Geometry check sheet. Reference: drawing and pictorial views, mm from the part's lowest x, y, z. A direction names the side the tool comes from. Give positions to 0.01 mm unless a question says otherwise; leave off trailing zeros. Write each loop counter-clockwise with the first axis right and the second up, starting at its lowest first coordinate (ties: lowest second). Pieces come first, ordered by that corner, then holes. Notation, with made-up numbers: M -29,70 L 30,70 A32 ccw 30,107 Z; hole C 1.25,-1 d11. An arc over 180 degrees is marked long. Write item = value, one per line. Start each with the question number.
1) Cross-section at A-A, the plane z = 10.25. Record the cut outline in (x, y) (3 decimals), plus the area to 3 significant figures.
2) Scan lines: line 1 along X through (y, z) = (7.25, 8); line 2 along Y through (x, z) = (7.5, 16.75); line 3 along X through (y, z) = (21.5, 6). Record each from-to range of solid material in increasing order. Write a range as [from, to].
3) Access from +Z, -Z, +X, -X, +Y, -Y to the whole of each face (thin tool, end or side, straight path). Record for the marked faces 4, 5 and 6.
4) Cross-section at B-B, the plane x = 12.5. Record the cut outline in (y, z), plus the area to 3 significant figures.
5) Mould release check, pull along X, two halves, no side actions. Record for the marked faces 1, 2 and 3: released by +X, released by -X, zero draft, split by the parting line, or undercut.
6) Cross-section at C-C, the plane y = 8.25. Give the number of separate pieces and of enclosed holes in the cut face, plus the area to 3 significant figures.
7) Go/stop test with flat-tipped pins: pin 1 (1.5 mm diameter, centred on y = 6, z = 15, fed in from -X); pin 2 (2 mm diameter, centred on y = 16.5, z = 8.5, fed in from -X); pin 3 (3 mm diameter, centred on y = 18.5, z = 5, fed in from -X). Record where each tip stops, or that it passes through.
8) Cross-section at D-D, the plane z = 4. Record the cut outline in (x, y) (3 decimals), plus the area to 3 significant figures.
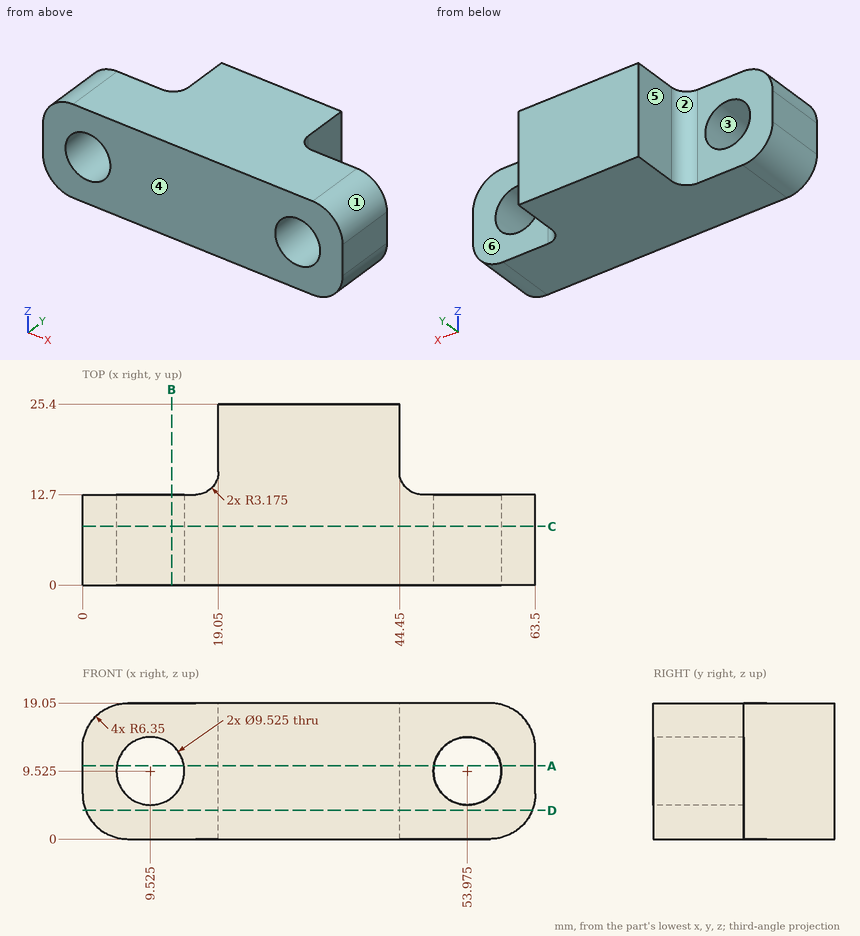
Reply:
q1.outline = M 0,0 L 4.818,0 L 4.818,12.7 L 0,12.7 Z; M 14.232,0 L 49.268,0 L 49.268,12.7 L 47.625,12.7 A3.175 cw 44.45,15.875 L 44.45,25.4 L 19.05,25.4 L 19.05,15.875 A3.175 cw 15.875,12.7 L 14.232,12.7 Z; M 58.682,0 L 63.5,0 L 63.5,12.7 L 58.682,12.7 Z
q1.area = 894 mm2
q2.line_1 = [0, 5.01], [14.04, 49.46], [58.49, 63.5]
q2.line_2 = [0, 12.7]
q2.line_3 = [19.05, 44.45]
q3.face_4 = +Z, -Z, +X, -X, -Y
q3.face_5 = +Z, -Z, -X, +Y
q3.face_6 = +Z, -Z, +X, +Y
q4.outline = M 0,0 L 12.7,0 L 12.7,5.81 L 0,5.81 Z; M 0,13.24 L 12.7,13.24 L 12.7,19.05 L 0,19.05 Z
q4.area = 147 mm2
q5.face_1 = released by +X
q5.face_2 = released by -X
q5.face_3 = undercut
q6.separate_pieces = 1
q6.enclosed_holes = 2
q6.area = 1,030 mm2
q7.pin_1 = 0.19
q7.pin_2 = 19.03
q7.pin_3 = 19.05
q8.outline = M 0.451,0 L 63.049,0 L 63.049,12.7 L 47.625,12.7 A3.175 cw 44.45,15.875 L 44.45,25.4 L 19.05,25.4 L 19.05,15.875 A3.175 cw 15.875,12.7 L 0.451,12.7 Z
q8.area = 1,120 mm2
